Source: CAD feature listing. Evaluate the final solid. Frame: model axes, mm. A direction names the side the tool comes from. Give positions to 0.01 mm unless a question says otherwise; leave off trailing zeros. Loops run counter-clockwise (first coordinate to the right, second up) from the corner with the lowest first, then second, coordinate; pieces in that order, holes last. Notation, with made-up numbers: (59, -14.75) -> (115, -14.75) arc R22 ccw to (115, 20.25) -> close; hole circle Ø3 at (79.25, 49). An arc over 180 degrees is marked (long way). Return JSON: item names as keys, results as strings. Group by question number.
```python
from build123d import *

# Parameters (mm, degrees)
F1_DEPTH = 38.1
F2_W     = 18.796
F2_H     = 38.1
F3_DEPTH = 127


with BuildPart() as f1:
    # F0 (on Top) → F1 (new body)
    with BuildSketch(Plane.XY):
        Polygon((38.974344, 14.27756), (-36.971656, 14.27756), (-36.971656, -4.51844), (-11.571656, -4.51844), (-11.571656, -17.11684), (13.574344, -17.11684), (13.574344, -4.51844), (38.974344, -4.51844), align=None)
    extrude(amount=F1_DEPTH)

    # F2 (on face) → F3 (join)
    with BuildSketch(Plane.YZ.offset(38.974344)):
        with Locations((4.87956, 19.05)):
            Rectangle(F2_W, F2_H)
    extrude(amount=F3_DEPTH)


solid = f1.part
```
1) Contact query for flat-ended pins moving along their axis: P1, Ø8, axis at x = 58, z = 6.5, coming from the -Y side; P2, Ø10, axis at y = -10, z = 17.5, coming from the -X side; P3, Ø4, axis at y = -11.5, z = 25.5, coming from the +X side. Output: stop coordinate, or through.
2) Material intervals for line 1 (Y direction, x = 108, z = 4.5); line 2 (X direction, y = -10.5, z = 24.5), sorted ascending.
3) Reachability of faces 1 (the face through (-24, -4.518, 19)), 2 (the face through (89, -4.518, 19)), 3 (the face through (63, 14.278, 19)) from +Z, -Z, +X, -X, +Y, -Y: full face, straight path, thin tool, end or side. Return the list, or none.
4) Cut plane B-B on y = -10.5. Return loops of the section in (x, z), then the cut area to 3 significant figures.
5) Cut plane A-A on z = 9.5. Return loops of the section in (x, y).
6) Cut plane C-C on x = 154.5. Return loops of the section in (y, z).
Calculated:
{
 "1": {"P1": "y = -4.52", "P2": "x = -11.57", "P3": "x = 13.57"},
 "2": {"line 1": "-4.52 to 14.28", "line 2": "-11.57 to 13.57"},
 "3": {"face 1": "+Z, -Z, -X, -Y", "face 2": "+Z, -Z, +X, -Y", "face 3": "+Z, -Z, +X, -X, +Y"},
 "4": {"outline": "(-11.57, 0) -> (13.57, 0) -> (13.57, 38.1) -> (-11.57, 38.1) -> close", "area": "958 mm2"},
 "5": {"outline": "(-36.97, -4.52) -> (-11.57, -4.52) -> (-11.57, -17.12) -> (13.57, -17.12) -> (13.57, -4.52) -> (165.97, -4.52) -> (165.97, 14.28) -> (-36.97, 14.28) -> close"},
 "6": {"outline": "(-4.52, 0) -> (14.28, 0) -> (14.28, 38.1) -> (-4.52, 38.1) -> close"}
}
